```python
from build123d import *

# Parameters (mm, degrees)
F1_DEPTH = 50.8
F2_W     = 17.4146303907
F2_H     = 14.1386073083
F3_DEPTH = 18.779527396


with BuildPart() as f1:
    # F0 (on Front) → F1 (new body)
    with BuildSketch(Plane.XZ):
        Polygon((0, 48.3591668308), (0, 0), (68.5028927401, 0), (68.5028927401, 48.3591668308), (51.0882623494, 48.3591668308), (51.0882623494, 29.5796394348), (17.4146303907, 29.5796394348), (17.4146303907, 48.3591668308), align=None)
    extrude(amount=F1_DEPTH)

    # F2 (on face) → F3 (cut, through all)
    with BuildSketch(Plane.XY.offset(48.3591668308)):
        with Locations((59.7955775447, -23.6191870645)):
            Rectangle(F2_W, F2_H)
    extrude(amount=-F3_DEPTH, mode=Mode.SUBTRACT)


solid = f1.part
```
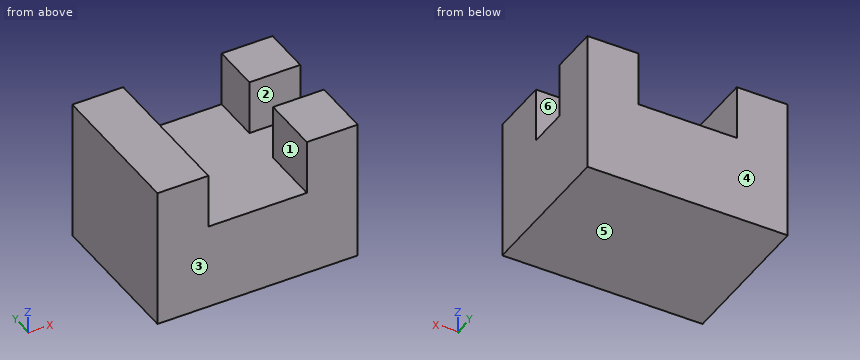
The model under review builds one solid part; all positions refer to its coordinate system, in mm. Face numbers are marked on the shaded views. A direction names the side the tool comes from. Round coordinates to 2 decimals unless told otherwise and drop trailing zeros. Order: outer loops, then holes, each group sorted by start corner. A loop starts at its lowest first (then second) coordinate and runs counter-clockwise, first axis right, second up. Notation, with made-up numbers: (6, 14.5) - (63, 14.5) arc R30 cw to (63, 51.5) - close; hole circle Ø10 at (44.25, -5). An arc over 180 degrees is marked (long way). Answer in a Markdown table with one row per item.
(1) For line 1 (X direction, y = -36, z = 34); line 2 (Y direction, x = 60, z = 45); line 3 (Z direction, x = 32, y = -19.5), list the stretches that pass through material, from the lowest coordinate up. Write a range as from..to.
Result set:
| item | result |
|---|---|
| line 1 | x = 0..17.41, 51.09..68.5 |
| line 2 | y = -50.8..-30.69, -16.55..0 |
| line 3 | z = 0..29.58 |
(2) Take a section at B-B on x = 61. Write out the cut boundary in (y, z), plus the area to 3 significant figures.
Result set:
| item | result |
|---|---|
| outline | (-50.8, 0) - (0, 0) - (0, 48.36) - (-16.55, 48.36) - (-16.55, 29.58) - (-30.69, 29.58) - (-30.69, 48.36) - (-50.8, 48.36) - close |
| area | 2,190 mm2 |
(3) Take a section at C-C on y = -33.5. Write out the cut boundary in (x, z), plus the area to 3 significant figures.
Result set:
| item | result |
|---|---|
| outline | (0, 0) - (68.5, 0) - (68.5, 48.36) - (51.09, 48.36) - (51.09, 29.58) - (17.41, 29.58) - (17.41, 48.36) - (0, 48.36) - close |
| area | 2,680 mm2 |
(4) Take a section at D-D on y = -20. Write out the cut boundary in (x, z).
Result set:
| item | result |
|---|---|
| outline | (0, 0) - (68.5, 0) - (68.5, 29.58) - (17.41, 29.58) - (17.41, 48.36) - (0, 48.36) - close |
(5) Machinability: for the marked faces 1, 2 and 3, which of the approach directions +Z, -Z, +X, -X, +Y, -Y give a long, thin tool a straight path to every point of the face, cutting with its end or side? Answer none if there is none.
Result set:
| item | result |
|---|---|
| face 1 | +Z, +Y, -Y |
| face 2 | +Z, +X |
| face 3 | +Z, -Z, +X, -X, -Y |
(6) Clearance check with a flat-ended pin moving along its axis: P1, Ø10, axis at x = 26, y = -28, coming from the +Z side. State where the tip first meets the part, or that it passes through.
Result set:
| item | result |
|---|---|
| P1 | stops at z = 29.58 |
(7) Take a section at A-A on z = 40.5. Write out the cut boundary in (x, y).
Result set:
| item | result |
|---|---|
| outline | (0, -50.8) - (17.41, -50.8) - (17.41, 0) - (0, 0) - close; (51.09, -50.8) - (68.5, -50.8) - (68.5, -30.69) - (51.09, -30.69) - close; (51.09, -16.55) - (68.5, -16.55) - (68.5, 0) - (51.09, 0) - close |
(8) Mouldability with a two-part tool opening along Y and no side actions: class the marked faces 4, 5 and 6 as released by +Y, released by -Y, zero draft, split by the parting line, or undercut.
Result set:
| item | result |
|---|---|
| face 4 | released by +Y |
| face 5 | zero draft |
| face 6 | undercut |
